Build history of the part. All positions in model axes, mm. Face numbers are marked on the shaded views. A direction names the side the tool comes from. Round coordinates to 2 decimals unless told otherwise and drop trailing zeros. Loops run counter-clockwise (first coordinate to the right, second up) from the corner with the lowest first, then second, coordinate; pieces in that order, holes last. Notation, with made-up numbers: M 49,61.25 L 54,61.25 A19 cw 54,88.25 Z; hole C 60,-14.75 d5. An arc over 180 degrees is marked long. Use one line per item in the form item = value. Start each with the question number.
```python
from build123d import *

# Parameters (mm, degrees)
PAD_DEPTH = 3.6
FILLET_R  = 0.4


with BuildPart() as part:
    # Sketch → Pad (new body, symmetric)
    with BuildSketch(Plane.XZ):
        Polygon((-5.7, 0), (5.7, 0), (5.7, 5.09), (4.56, 5.09), (4.56, 1.15), (2.29, 1.15), (2.29, 5.09), (1.15, 5.09), (1.15, 1.15), (-1.15, 1.15), (-1.15, 5.09), (-2.29, 5.09), (-2.29, 1.15), (-4.56, 1.15), (-4.56, 5.09), (-5.7, 5.09), align=None)
    extrude(amount=PAD_DEPTH, both=True)

    # Fillet
    fillet_edges = [part.edges().sort_by_distance(p)[0] for p in [
        (-5.7, 0, 5.09),
        (-4.56, 0, 5.09),
        (-2.29, 0, 5.09),
        (-1.15, 0, 5.09),
        (1.15, 0, 5.09),
        (2.29, 0, 5.09),
        (4.56, 0, 5.09),
        (5.7, 0, 5.09),
        (-4.56, 0, 1.15),
        (-1.15, 0, 1.15),
        (2.29, 0, 1.15),
        (-2.29, 0, 1.15),
        (1.15, 0, 1.15),
        (4.56, 0, 1.15),
    ]]
    fillet(fillet_edges, radius=FILLET_R)


solid = part.part
```
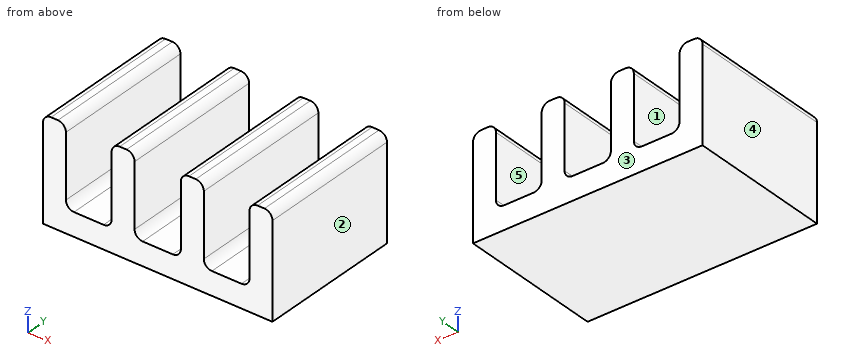
Q1. Saw through at C-C (x = 3.5). Give the cut face in (y, z).
Q2. Saw through at D-D (x = -2.5). Give the cut face in (y, z).
Q3. Drop flat-ended pins along their axis: P1, Ø0.7, axis at x = -3.5, y = -0.5, coming from the +Z side; P2, Ø1.6, axis at x = 0.5, y = -1.5, coming from the +Z side. Give the stop position or say it passes through.
Q4. Saw through at A-A (z = 3.25). Give the cut face in (x, y).
Q5. Wall check: probe 1 along X at (y, z) = (1, 3); probe 2 along Z at (x, y) = (0.25, 0.75); probe 3 along Z at (x, y) = (-1.5, 0). Give the ranges that are in metal, low to high.
Q6. Pull direction X, two halves, no side cores. Call the marked faces 1, 2 and 3: pulls with the +X half, pulls with the -X half, needs draft (parallel to the pull), parting line crosses it, or undercut.
Q7. Tool access for the marked faces 4 and 5: list every direction of +Z, -Z, +X, -X, +Y, -Y with a clear straight run to the whole face (end or side of a thin tool).
Filled in:
q1.outline = M -3.6,0 L 3.6,0 L 3.6,1.15 L -3.6,1.15 Z
q2.outline = M -3.6,0 L 3.6,0 L 3.6,1.2 L -3.6,1.2 Z
q3.P1 = 1.15
q3.P2 = 5
q4.outline = M -5.7,-3.6 L -4.56,-3.6 L -4.56,3.6 L -5.7,3.6 Z; M -2.29,-3.6 L -1.15,-3.6 L -1.15,3.6 L -2.29,3.6 Z; M 1.15,-3.6 L 2.29,-3.6 L 2.29,3.6 L 1.15,3.6 Z; M 4.56,-3.6 L 5.7,-3.6 L 5.7,3.6 L 4.56,3.6 Z
q5.probe_1 = -5.7 to -4.56, -2.29 to -1.15, 1.15 to 2.29, 4.56 to 5.7
q5.probe_2 = 0 to 1.15
q5.probe_3 = 0 to 5.09
q6.face_1 = undercut
q6.face_2 = pulls with the +X half
q6.face_3 = needs draft
q7.face_4 = +Z, -Z, -X, +Y, -Y
q7.face_5 = +Z, +Y, -Y
